Input: part model. Units: mm. Frame: model coordinates. A direction names the side the tool comes from. Give positions to 0.01 mm unless a question says otherwise; leave off trailing zeros. Loops run counter-clockwise (first coordinate to the right, second up) from the corner with the lowest first, then second, coordinate; pieces in that order, holes last. Notation, with made-up numbers: M 32.25,-21 L 91.25,-21 A19 ccw 91.25,1 Z; hole C 74,61 d6. An arc over 180 degrees is marked long. One line per item, written item: value. Start each with the question number.
(1) Section B-B on z = 19.25. Output: boundary loops of the cut face in (x, y), plus the area to 3 significant figures.
(2) Section C-C on x = 25.8. Output: boundary loops of the cut face in (y, z), plus the area to 3 significant figures.
(3) Ray query, line 1 along X through (y, z) = (3.25, 19.25); line 2 along Z through (x, y) = (25.8, 2); line 3 along X through (y, z) = (3.5, 7). Return the intervals inside material, ascending. Write a range as from..to.
(4) Access query for faces 5 (the flat face through (-15, 2, 10)), 6 (the flat face through (20, 3.5, -2)), 7 (the flat face through (20, 0, 11)). Directions: +Z, -Z, +X, -X, +Y, -Y. A direction counts if a zero-diameter tool reaches every point of the face in a straight line with its end or side. Return the directions, or none.
(5) Pin query (flat end, axial travel): P1, Ø1.8, axis at x = 19, y = 1, coming from the -Z side; P2, Ø0.8, axis at x = -24.5, z = -2.5, coming from the -Y side; P3, Ø7.5, axis at x = -5, z = 5.5, coming from the -Y side. Return the tip coordinate at first contact, or that it passes through.
(6) Section A-A on y = 2.75. Output: boundary loops of the cut face in (x, z).
(7) Section D-D on z = 3.75. Output: boundary loops of the cut face in (x, y), plus the area to 4 significant figures.
(8) Pull-direction query (Z, two-part tool) for faces 1 (the flat face through (-22, 3.5, -2)), 2 (the flat face through (0, 6, -3.75)), 3 (the flat face through (0, 6, 23.25)), 4 (the cylindrical face through (-23.966, 3.895, 17.465)); classes: released by +Z, released by -Z, zero draft, split by the parting line, or undercut.
```python
from build123d import *

# Parameters (mm, degrees)
SKETCH1_W                  = 60
SKETCH1_H                  = 2.5
BOSS_EXTRUDE1_DEPTH        = 2.5
SKETCH2_W                  = 60
SKETCH2_H                  = 5
BOSS_EXTRUDE2_DEPTH        = 3
SKETCH5_W                  = 60
SKETCH5_H                  = 5.5
BOSS_EXTRUDE4_DEPTH        = 22
SKETCH6_W                  = 60
SKETCH6_H                  = 27
BOSS_EXTRUDE5_DEPTH        = 2.4
F_3_6_3_6_DIAMETER_HOLE1_D = 3.6
SKETCH9_W                  = 25
SKETCH9_H                  = 9.609635329
CUT_EXTRUDE1_DEPTH         = 42.126755282
SKETCH10_W                 = 60
SKETCH10_H                 = 3.5
CUT_EXTRUDE2_DEPTH         = 40.530494558


with BuildPart() as part:
    # Sketch1 → Boss-Extrude1 (new body)
    with BuildSketch(Plane(origin=(0, 0, 0), x_dir=(1, 0, 0), z_dir=(0, 1, 0))):
        Rectangle(SKETCH1_W, SKETCH1_H)
    extrude(amount=BOSS_EXTRUDE1_DEPTH)

    # Sketch2 → Boss-Extrude2 (add)
    with BuildSketch(Plane(origin=(0, 2.5, 0), x_dir=(1, 0, 0), z_dir=(0, 1, 0))):
        with Locations((0, 1.25)):
            Rectangle(SKETCH2_W, SKETCH2_H)
    extrude(amount=BOSS_EXTRUDE2_DEPTH)

    # Sketch5 → Boss-Extrude4 (add)
    with BuildSketch(Plane.XY.offset(1.25)):
        with Locations((0, 2.75)):
            Rectangle(SKETCH5_W, SKETCH5_H)
    extrude(amount=BOSS_EXTRUDE4_DEPTH)

    # Sketch6 → Boss-Extrude5 (add)
    with BuildSketch(Plane(origin=(0, 5.5, 0), x_dir=(1, 0, 0), z_dir=(0, 1, 0))):
        with Locations((0, -9.75)):
            Rectangle(SKETCH6_W, SKETCH6_H)
    extrude(amount=BOSS_EXTRUDE5_DEPTH)

    # Ø3.6 (3.6) Diameter Hole1 (through all)
    with Locations(Plane(origin=(0, 7.9, 0), x_dir=(1, 0, 0), z_dir=(0, 1, 0))):
        with Locations((-24.2, -19.25), (25.8, -19.25)):
            Hole(F_3_6_3_6_DIAMETER_HOLE1_D / 2)

    # Sketch9 → Cut-Extrude1 (cut, through all)
    with BuildSketch(Plane(origin=(0, 0, -3.75), x_dir=(-1, 0, 0), z_dir=(0, 0, -1))):
        with Locations((2.5, 0.095182336)):
            Rectangle(SKETCH9_W, SKETCH9_H)
    extrude(amount=-CUT_EXTRUDE1_DEPTH, mode=Mode.SUBTRACT)

    # Sketch10 → Cut-Extrude2 (cut, through all)
    with BuildSketch(Plane(origin=(0, 0, -1.25), x_dir=(-1, 0, 0), z_dir=(0, 0, -1))):
        with Locations((0, 1.75)):
            Rectangle(SKETCH10_W, SKETCH10_H)
    extrude(amount=CUT_EXTRUDE2_DEPTH, mode=Mode.SUBTRACT)


solid = part.part
```
Output values:
1. outline: M -30,0 L -26,0 L -26,7.9 L -30,7.9 Z; M -22.4,0 L -15,0 L -15,4.9 L 10,4.9 L 10,0 L 24,0 L 24,7.9 L -22.4,7.9 Z; M 27.6,0 L 30,0 L 30,7.9 L 27.6,7.9 Z
1. area: 295 mm²
2. outline: M 0,-1.25 L 3.5,-1.25 L 3.5,-3.75 L 7.9,-3.75 L 7.9,17.45 L 0,17.45 Z; M 0,21.05 L 7.9,21.05 L 7.9,23.25 L 0,23.25 Z
2. area: 176 mm²
3. line 1: x = -30..-26, -22.4..-15, 10..24, 27.6..30
3. line 2: z = -1.25..17.45, 21.05..23.25
3. line 3: x = -30..-15, 10..30
4. face 5: +Z, -Z, -Y
4. face 6: -Z, +X, -X, -Y
4. face 7: +Z, -Z, +X, -X, -Y
5. P1: stops at z = -1.25
5. P2: stops at y = 3.5
5. P3: stops at y = 4.9
6. outline: M -30,-1.25 L -15,-1.25 L -15,23.25 L -30,23.25 Z; M 10,-1.25 L 30,-1.25 L 30,23.25 L 10,23.25 Z; hole C -24.2,19.25 d3.6; hole C 25.8,19.25 d3.6
7. outline: M -30,0 L -15,0 L -15,4.9 L 10,4.9 L 10,0 L 30,0 L 30,7.9 L -30,7.9 Z
7. area: 351.5 mm²
8. face 1: zero draft
8. face 2: released by -Z
8. face 3: released by +Z
8. face 4: undercut
